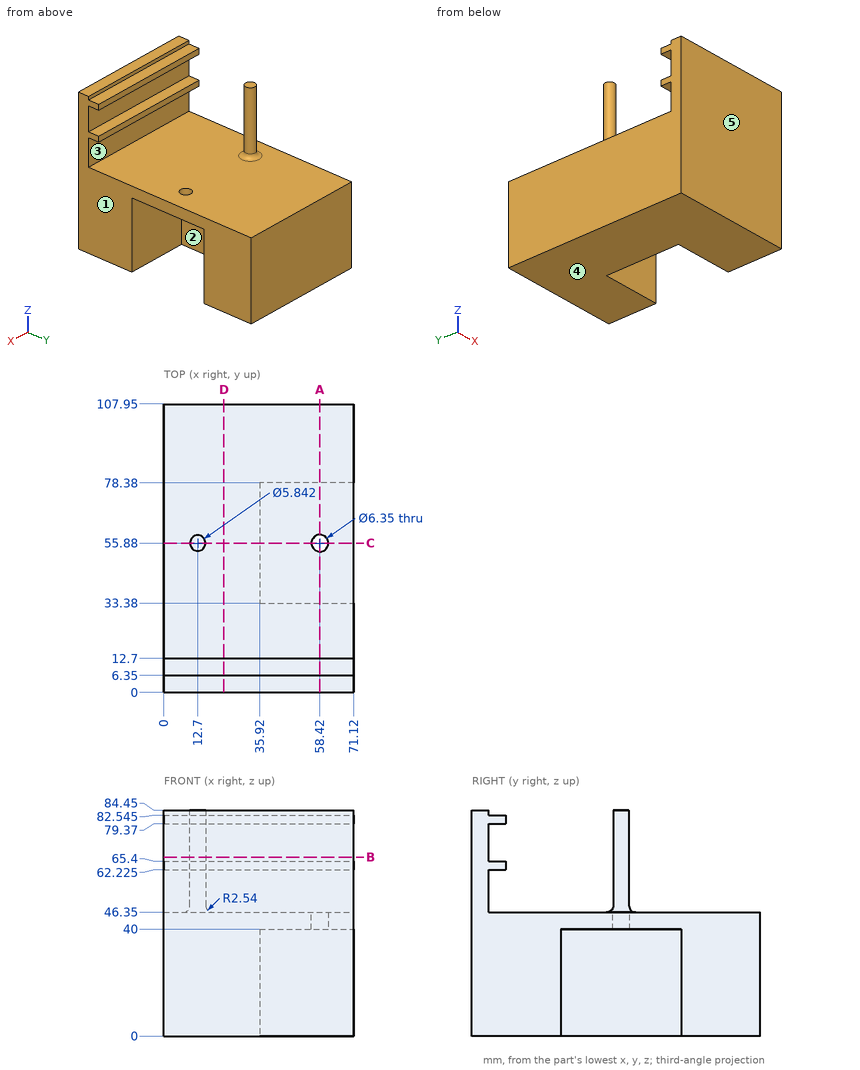
Could you check a few things on this drawing? It's one solid part, dimensions in mm from its lowest x, y, z. A direction names the side the tool comes from. Round coordinates to 2 decimals unless told otherwise and drop trailing zeros. Order: outer loops, then holes, each group sorted by start corner. A loop starts at its lowest first (then second) coordinate and runs counter-clockwise, first axis right, second up.
(1) Imagine slicing it at D-D (x = 22.5). Write out the boundary of the cut face in (y, z) (3 decimals), plus the area to 3 significant figures.
Response values:
outline: (0, 0) - (107.95, 0) - (107.95, 46.35) - (6.35, 46.35) - (6.35, 62.225) - (12.7, 62.225) - (12.7, 65.4) - (6.35, 65.4) - (6.35, 79.37) - (12.7, 79.37) - (12.7, 82.545) - (6.35, 82.545) - (6.35, 84.45) - (0, 84.45) - close
area: 5,290 mm2
(2) Please list where these lines run through material, in increasing order: line 1 along Y through (x, z) = (58.42, 44.25) (3 decimals); line 2 along Y through (x, z) = (59.5, 31); line 3 along Y through (x, z) = (44.5, 80).
Response values:
line 1: y = 0 to 52.705, 59.055 to 107.95
line 2: y = 0 to 33.38, 78.38 to 107.95
line 3: y = 0 to 12.7
(3) Imagine slicing it at B-B (z = 67). Write out the boundary of the cut face in (x, y), plus the area to 3 significant figures.
Response values:
outline: (0, 0) - (71.12, 0) - (71.12, 6.35) - (0, 6.35) - close; circle Ø5.84 at (12.7, 55.88)
area: 478 mm2
(4) I'm going to push flat-ended pins straight in: pin 1 (4 mm diameter, centred on x = 16, y = 94, fed in from +Z); pin 2 (8 mm diameter, centred on y = 45.5, z = 66.5, fed in from +X); pin 3 (7 mm diameter, centred on x = 34, z = 75, fed in from +Y); pin 4 (2.5 mm diameter, centred on x = 45.5, z = 81, fed in from +Y). Where does each tip first touch, or does it pass through?
Response values:
pin 1: stops at z = 46.35
pin 2: passes through
pin 3: stops at y = 6.35
pin 4: stops at y = 12.7
(5) Imagine slicing it at C-C (y = 55.88). Write out the boundary of the cut face in (x, z) (3 decimals).
Response values:
outline: (0, 0) - (35.92, 0) - (35.92, 40) - (55.245, 40) - (55.245, 46.35) - (18.161, 46.35) arc R2.54 cw to (15.621, 48.89) - (15.621, 84.45) - (9.779, 84.45) - (9.779, 48.89) arc R2.54 cw to (7.239, 46.35) - (0, 46.35) - close; (61.595, 40) - (71.12, 40) - (71.12, 46.35) - (61.595, 46.35) - close
(6) Which directions (+Z, -Z, +X, -X, +Y, -Y) give clear straight access to the entire face, cutting with the end or side of a thin tool? Please do the marked faces 1 and 2.
Response values:
face 1: +Z, -Z, +X, +Y, -Y
face 2: -Z, +X
(7) Imagine slicing it at A-A (x = 58.42). Write out the boundary of the cut face in (y, z) (3 decimals), plus the area to 3 significant figures.
Response values:
outline: (0, 0) - (33.38, 0) - (33.38, 40) - (52.705, 40) - (52.705, 46.35) - (6.35, 46.35) - (6.35, 62.225) - (12.7, 62.225) - (12.7, 65.4) - (6.35, 65.4) - (6.35, 79.37) - (12.7, 79.37) - (12.7, 82.545) - (6.35, 82.545) - (6.35, 84.45) - (0, 84.45) - close; (59.055, 40) - (78.38, 40) - (78.38, 0) - (107.95, 0) - (107.95, 46.35) - (59.055, 46.35) - close
area: 3,450 mm2
(8) If we mould it in two halves opening along Z, with no side actions, what happens to the marked faces 3, 4 and 5? For each: released by +Z, released by -Z, zero draft, split by the parting line, or undercut.
Response values:
face 3: undercut
face 4: released by -Z
face 5: zero draft
